Geometry check sheet. Reference: drawing and pictorial views, mm from the part's lowest x, y, z. Give positions to 0.01 mm unless a question says otherwise; leave off trailing zeros. Order: outer loops, then holes, each group sorted by start corner. A loop starts at its lowest first (then second) coordinate and runs counter-clockwise, first axis right, second up.
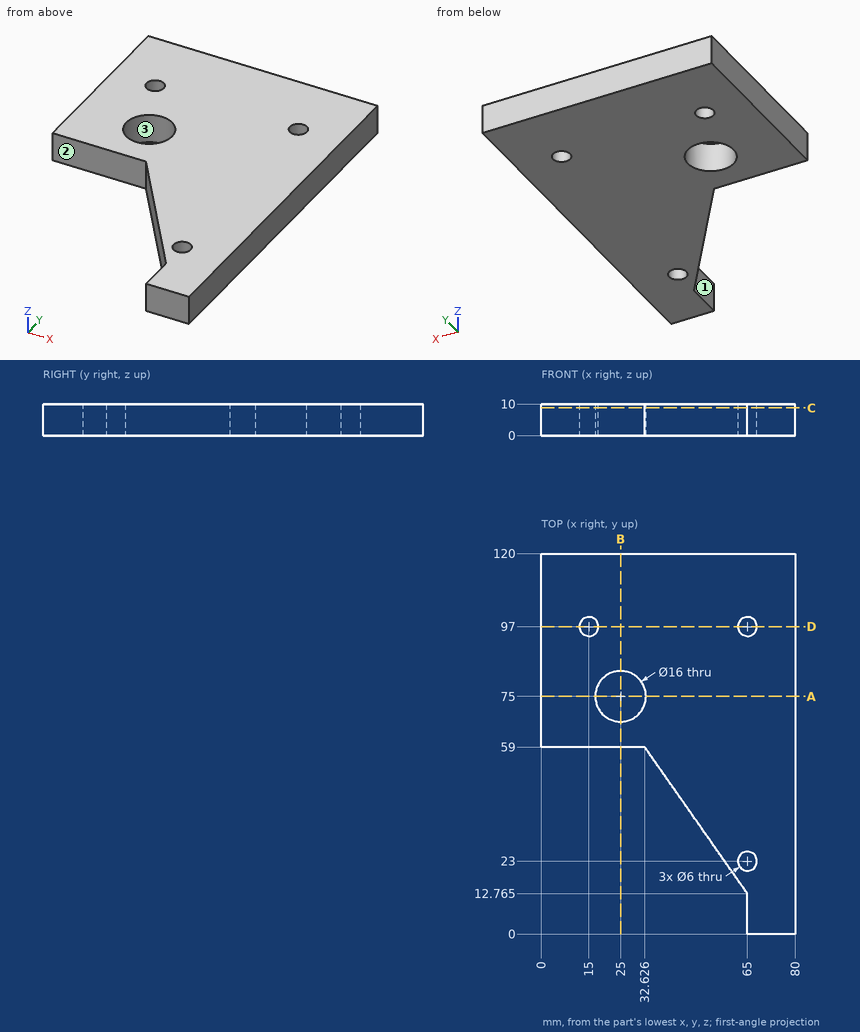
(1) Sectioned sample at B-B (x = 25). Enter the section's corners in (y, z), plus the area to 3 significant figures.
(2) Sectioned sample at D-D (y = 97). Enter the section's corners in (x, z).
(3) Thickness scan on L1, parallel to Y at x = 67, z = 4.5 (1 decimal); L2, parallel to Y at x = 25, z = 3; L3, parallel to Y at x = 63.5, z = 6.75 (1 decimal). Record the ranges inside material, lowest first.
(4) Sectioned sample at C-C (z = 8.75). Enter the section's corners in (x, y) (1 decimal), plus the area to 3 significant figures.
(5) Release check for a two-part mould opening along Y. For the marked faces 1, 2 and 3 record: released by +Y, released by -Y, zero draft, split by the parting line, or undercut.
(6) Sectioned sample at A-A (y = 75). Enter the section's corners in (x, z), plus the area to 3 significant figures.
(7) Go/stop test with flat-tipped pins: P1, Ø18.5, axis at x = 25, y = 75, coming from the -Z side; P2, Ø5, axis at y = 41, z = 6.5, coming from the -X side; P3, Ø3, axis at y = 8, z = 6, coming from the -X side; P4, Ø4, axis at x = 62, z = 6.5, coming from the -Y side. Record where each tip stops, or that it passes through.
Values follow:
1. outline: (59, 0) - (67, 0) - (67, 10) - (59, 10) - close; (83, 0) - (120, 0) - (120, 10) - (83, 10) - close
1. area: 450 mm2
2. outline: (0, 0) - (12, 0) - (12, 10) - (0, 10) - close; (18, 0) - (62, 0) - (62, 10) - (18, 10) - close; (68, 0) - (80, 0) - (80, 10) - (68, 10) - close
3. L1: y = 0 to 20.8, 25.2 to 94.8, 99.2 to 120
3. L2: y = 59 to 67, 83 to 120
3. L3: y = 14.9 to 20.4, 25.6 to 94.4, 99.6 to 120
4. outline: (0, 59) - (32.6, 59) - (65, 12.8) - (65, 0) - (80, 0) - (80, 120) - (0, 120) - close; hole circle Ø6 at (15, 97); hole circle Ø16 at (25, 75); hole circle Ø6 at (65, 23); hole circle Ø6 at (65, 97)
4. area: 6,230 mm2
5. face 1: zero draft
5. face 2: released by -Y
5. face 3: undercut
6. outline: (0, 0) - (17, 0) - (17, 10) - (0, 10) - close; (33, 0) - (80, 0) - (80, 10) - (33, 10) - close
6. area: 640 mm2
7. P1: stops at z = 0
7. P2: stops at x = 43.48
7. P3: stops at x = 65
7. P4: stops at y = 14.19
